Here's how the part is built. I have some questions about the finished solid (model axes, mm). A direction names the side the tool comes from. Coordinates: 2 decimals unless noted, no trailing zeros. Order: outer loops, then holes, each group sorted by start corner. A loop starts at its lowest first (then second) coordinate and runs counter-clockwise, first axis right, second up. Notation, with made-up numbers: (27.5, -30) - (37.5, -30) arc R29 ccw to (37.5, 3) - close; hole circle Ø5 at (20.25, 44). An arc over 180 degrees is marked (long way). Use CSV: the item, a comma, the result in double quotes. Start each with the question number.
from build123d import *

# Parameters (mm, degrees)
SKETCH1_W           = 152.4
SKETCH1_H           = 101.6
BOSS_EXTRUDE1_DEPTH = 127
CUT_EXTRUDE1_DEPTH  = 134.62
CUT_EXTRUDE2_DEPTH  = 134.62
SKETCH5_W           = 101.732493014
SKETCH5_H           = 12.7
CUT_EXTRUDE4_DEPTH  = 50.8


with BuildPart() as part:
    # Sketch1 → Boss-Extrude1 (new body)
    with BuildSketch(Plane.XY):
        with Locations((-47.482496627, -19.988512007)):
            Rectangle(SKETCH1_W, SKETCH1_H)
    extrude(amount=-BOSS_EXTRUDE1_DEPTH)

    # Sketch2 → Cut-Extrude1 (cut)
    with BuildSketch(Plane(origin=(0, 0, 0), x_dir=(0, 0, -1), z_dir=(1, 0, 0))):
        Polygon((0, 30.811487993), (0, -32.688512007), (63.5, 30.811487993), align=None)
    extrude(amount=CUT_EXTRUDE1_DEPTH, mode=Mode.SUBTRACT)

    # Sketch3 → Cut-Extrude2 (cut)
    with BuildSketch(Plane(origin=(0, 0, 0), x_dir=(0, 0, -1), z_dir=(1, 0, 0))):
        Polygon((0, -32.688512007), (0, 30.811487993), (63.5, 30.811487993), align=None)
    extrude(amount=-CUT_EXTRUDE2_DEPTH, mode=Mode.SUBTRACT)

    # Sketch5 → Cut-Extrude4 (cut)
    with BuildSketch(Plane(origin=(0, 28.105743997, -28.105743997), x_dir=(1, 0, 0), z_dir=(0, -0.7071067811865512, 0.7071067811865438))):
        with Locations((-47.548743134, -29.464268507)):
            Rectangle(SKETCH5_W, SKETCH5_H)
    extrude(amount=CUT_EXTRUDE4_DEPTH, mode=Mode.SUBTRACT)


solid = part.part
Item 1: Suppose I cut it at C-C on y = -1.5. Write out the boundary of the cut face in (x, z), then the cut area to 3 significant figures.
Item 2: Suppose I cut it at B-B on y = -30. Write out the boundary of the cut face in (x, z), then the cut area to 3 significant figures.
Item 3: Suppose I cut it at A-A on x = -85. Write out the boundary of the cut face in (y, z).
Item 4: Suppose I cut it at D-D on x = -100.5. Write out the boundary of the cut face in (y, z), then the cut area to 3 significant figures.
Item 5: Please list where these lines run through material, in increasing order: line 1 along X through (y, z) = (-14.5, -36); line 2 along Z through (x, y) = (-44, -33); line 3 along Z through (x, y) = (-49, -26). Write a range as from..to.
Item 6: For faces 1 (the flat face through (-123.682, -21, -77)), 2 (the flat face through (-48.26, -28.59, -12.96)), 3 (the flat face through (3.318, -11, -31)), which set-ups out of +Z, -Z, +X, -X, +Y, -Y let a thin tool reach every point of the face, with its end or its side?
Item 7: We'd pull the mould along Y, two halves only. Please class faces 4 (the flat face through (-49, -70.789, -63)), 5 (the flat face through (-48.26, -14.93, -35.72)), 6 (the flat face through (-48.26, 7.33, -48.88)), 7 (the flat face through (28.718, -21, -77)): released by +Y, released by -Y, zero draft, split by the parting line, or undercut.
Here are the results:
1,outline,"(-123.68, -127) - (28.72, -127) - (28.72, -31.19) - (3.32, -31.19) - (3.32, -49.15) - (-98.41, -49.15) - (-98.41, -31.19) - (-123.68, -31.19) - close"
1,area,"12,800 mm^2"
2,outline,"(-123.68, -127) - (28.72, -127) - (28.72, -2.69) - (-123.68, -2.69) - close; hole (-98.41, -20.65) - (3.32, -20.65) - (3.32, -14.37) - (-98.41, -14.37) - close"
2,area,"18,300 mm^2"
3,outline,"(-70.79, -127) - (30.81, -127) - (30.81, -63.5) - (11.76, -44.45) - (2.78, -53.43) - (-33.14, -17.51) - (-24.16, -8.53) - (-32.69, 0) - (-70.79, 0) - close"
4,outline,"(-70.79, -127) - (30.81, -127) - (30.81, -63.5) - (-32.69, 0) - (-70.79, 0) - close"
4,area,"10,900 mm^2"
5,line 1,"-123.68..-98.41, 3.32..28.72"
5,line 2,"-127..-17.65, -17.37..0"
5,line 3,"-127..-24.65, -10.37..-6.69"
6,face 1,"+Z, -Z, -X, +Y, -Y"
6,face 2,"+Y"
6,face 3,"none"
7,face 4,"released by -Y"
7,face 5,"undercut"
7,face 6,"undercut"
7,face 7,"zero draft"
